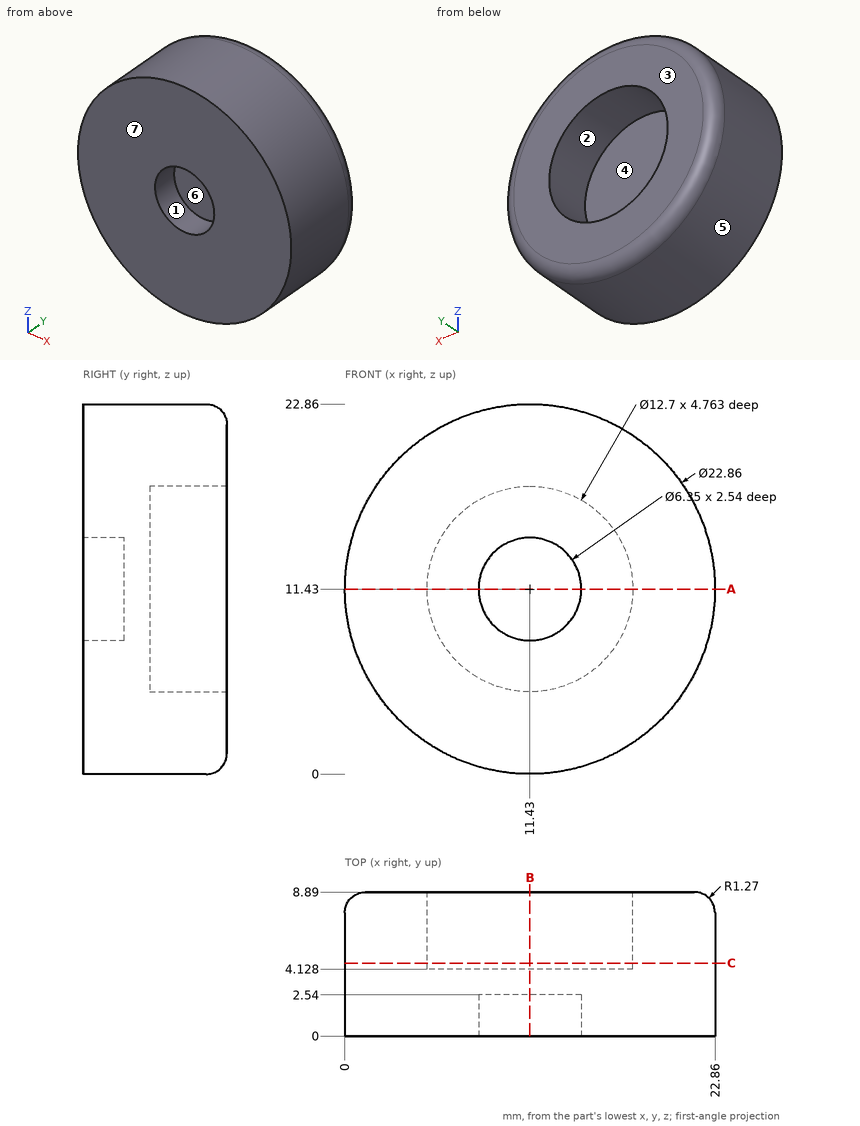
Verification items for this drawing (mm, ordinates from the low corner). A direction names the side the tool comes from. Give positions to 0.01 mm unless a question says otherwise; leave off trailing zeros. Loops run counter-clockwise (first coordinate to the right, second up) from the corner with the lowest first, then second, coordinate; pieces in that order, holes last. Notation, with made-up numbers: M 45.25,-30 L 97.25,-30 A10 ccw 97.25,-20 Z; hole C -35.5,-8 d6. An arc over 180 degrees is marked long. Answer as a JSON object with one key per item and string values. Group by question number.
Item 1: Access from +Z, -Z, +X, -X, +Y, -Y to the whole of each face (thin tool, end or side, straight path). Record for the marked faces 1, 2 and 3.
Item 2: Mould release check, pull along Z, two halves, no side actions. Record for the marked faces 4, 5, 6 and 7: pulls with the +Z half, pulls with the -Z half, needs draft (parallel to the pull), parting line crosses it, or undercut.
Item 3: Gauge pin test, flat ends, axial feed: pin 1 (8 mm diameter, centred on x = 14, z = 14, fed in from +Y); pin 2 (1 mm diameter, centred on x = 14.5, y = 4.5, fed in from -Z); pin 3 (1.5 mm diameter, centred on y = 3.5, z = 16, fed in from +X); pin 4 (1.9 mm diameter, centred on x = 12, z = 11.5, fed in from -Y). Record the tip position at first contact, or that the pin passes through.
Item 4: Sectioned sample at A-A on z = 11.43. Record the boundary of the cut face in (x, y) (1 decimal).
Item 5: Material ranges on L1, parallel to X at y = 2, z = 11.5 (1 decimal); L2, parallel to X at y = 5.5, z = 11.43; L3, parallel to Y at x = 15, z = 11.5, recorded low to high.
Item 6: Sectioned sample at B-B on x = 11.43. Record the boundary of the cut face in (y, z) (1 decimal).
Item 7: Sectioned sample at C-C on y = 4.5. Record the boundary of the cut face in (x, z).
Findings below:
{
 "1": {"face 1": "-Y", "face 2": "+Y", "face 3": "+Z, -Z, +X, -X, +Y"},
 "2": {"face 4": "undercut", "face 5": "parting line crosses it", "face 6": "undercut", "face 7": "needs draft"},
 "3": {"pin 1": "y = 8.89", "pin 2": "z = 0.29", "pin 3": "x = 22.2", "pin 4": "y = 2.54"},
 "4": {"outline": "M 0,0 L 8.3,0 L 8.3,2.5 L 14.6,2.5 L 14.6,0 L 22.9,0 L 22.9,7.6 A1.3 ccw 21.6,8.9 L 17.8,8.9 L 17.8,4.1 L 5.1,4.1 L 5.1,8.9 L 1.3,8.9 A1.3 ccw 0,7.6 Z"},
 "5": {"L1": "0 to 8.3, 14.6 to 22.9", "L2": "0 to 5.08, 17.78 to 22.86", "L3": "0 to 4.13"},
 "6": {"outline": "M 0,0 L 7.6,0 A1.3 ccw 8.9,1.3 L 8.9,5.1 L 4.1,5.1 L 4.1,17.8 L 8.9,17.8 L 8.9,21.6 A1.3 ccw 7.6,22.9 L 0,22.9 L 0,14.6 L 2.5,14.6 L 2.5,8.3 L 0,8.3 Z"},
 "7": {"outline": "C 11.43,11.43 d22.86; hole C 11.43,11.43 d12.7"}
}
